Check sheet for the drawn part. Datum: minimum x, y, z corner. Units: mm. A direction names the side the tool comes from. Give positions to 0.01 mm unless a question says otherwise; leave off trailing zeros. Loops run counter-clockwise (first coordinate to the right, second up) from the corner with the lowest first, then second, coordinate; pieces in that order, holes last.
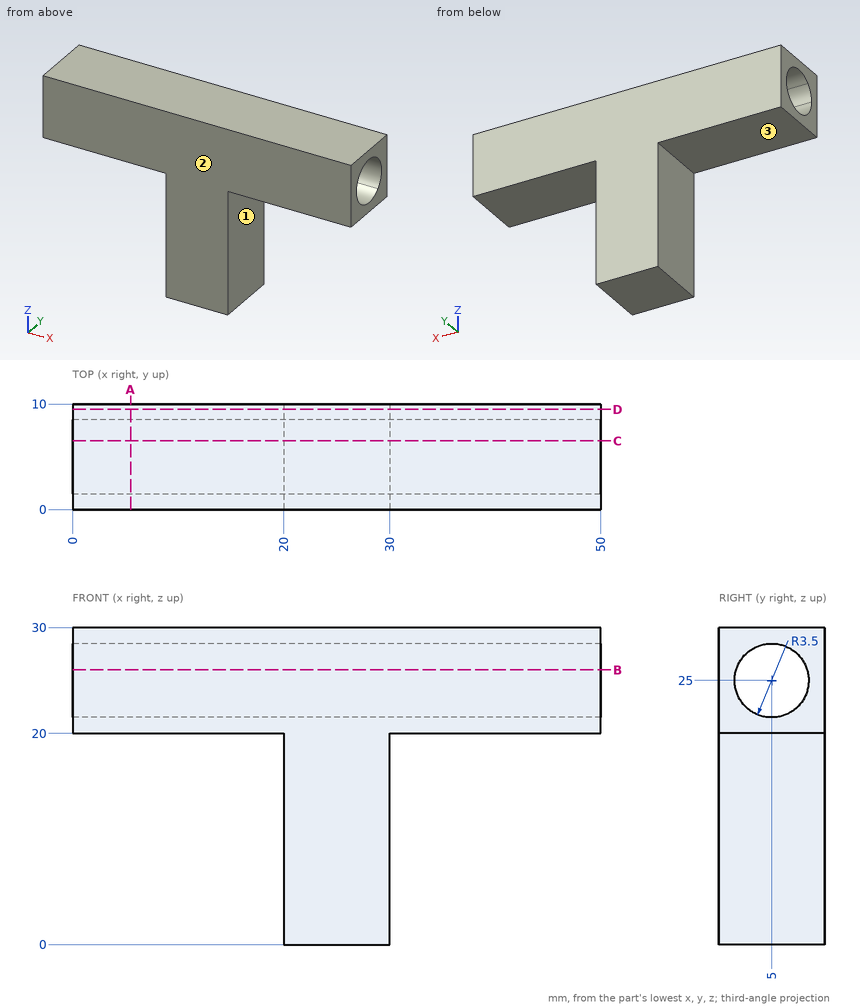
(1) Section check C-C on y = 6.5. Record the boundary of the cut face in (x, z).
(2) Access from +Z, -Z, +X, -X, +Y, -Y to the whole of each face (thin tool, end or side, straight path). Record for the marked faces 1, 2 and 3.
(3) Section check A-A on x = 5.5. Record the boundary of the cut face in (y, z).
(4) Section check B-B on z = 26. Record the boundary of the cut face in (x, y).
(5) Section check D-D on y = 9.5. Record the boundary of the cut face in (x, z), plus the area to 3 significant figures.
(6) Gauge pin test, flat ends, axial feed: pin 1 Ø3 at (x, y) = (10, 7.5) entering from -Z; pin 2 Ø3 at (y, z) = (4.5, 14) entering from -X; pin 3 Ø1.5 at (x, z) = (13, 17.5) entering from -Y. Record the tip position at first contact, or that the pin passes through.
(7) Material ranges on line 1 (Y direction, x = 37.5, z = 25); line 2 (Z direction, x = 42.5, y = 7); line 3 (X direction, y = 1.25, z = 6.5), recorded low to high.
Computed values:
1. outline: (0, 20) - (20, 20) - (20, 0) - (30, 0) - (30, 20) - (50, 20) - (50, 21.84) - (0, 21.84) - close; (0, 28.16) - (50, 28.16) - (50, 30) - (0, 30) - close
2. face 1: -Z, +X, +Y, -Y
2. face 2: +Z, -Z, +X, -X, -Y
2. face 3: -Z, -X, +Y, -Y
3. outline: (0, 20) - (10, 20) - (10, 30) - (0, 30) - close; hole (1.5, 25) arc R3.5 ccw (long way) to (2.53, 27.47) arc R3.5 ccw to start
4. outline: (0, 0) - (50, 0) - (50, 1.65) - (0, 1.65) - close; (0, 8.35) - (50, 8.35) - (50, 10) - (0, 10) - close
5. outline: (0, 20) - (20, 20) - (20, 0) - (30, 0) - (30, 20) - (50, 20) - (50, 30) - (0, 30) - close
5. area: 700 mm2
6. pin 1: stops at z = 20
6. pin 2: stops at x = 20
6. pin 3: passes through
7. line 1: y = 0 to 1.5, 8.5 to 10
7. line 2: z = 20 to 22.13, 27.87 to 30
7. line 3: x = 20 to 30
